from build123d import *

# Parameters (mm, degrees)
SKETCH_1_W                       = 78
SKETCH_1_H                       = 20
SM_BASE_FLANGE_1_DEPTH           = 1.5
SM_EDGE_FLANGE_1_STRIP_W         = 7.4732
SM_EDGE_FLANGE_1_STRIP_H         = 1.5
SM_EDGE_FLANGE_1_STRIP_CUT_DEPTH = 20
SM_EDGE_FLANGE_1_DEPTH           = 20
SM_EDGE_FLANGE_2_STRIP_W         = 7.4732
SM_EDGE_FLANGE_2_STRIP_H         = 1.5
SM_EDGE_FLANGE_2_STRIP_CUT_DEPTH = 20
SM_EDGE_FLANGE_2_DEPTH           = 20


# Sheet-metal steps are written as plain solids
with BuildPart() as part:
    # Sketch 1 → Базовая кромка1 (new body)
    with BuildSketch(Plane(origin=(0, 0, 0), x_dir=(1, 0, 0), z_dir=(0, 1, 0))):
        with Locations((39, 10)):
            Rectangle(SKETCH_1_W, SKETCH_1_H)
    extrude(amount=-SM_BASE_FLANGE_1_DEPTH)

    # Ребро-кромка1 strip (across the edge) → Ребро-кромка1 strip cut (cut)
    with BuildSketch(Plane.XY.offset(-20)):
        with Locations((-1.5, -0.75)):
            Rectangle(SM_EDGE_FLANGE_1_STRIP_W, SM_EDGE_FLANGE_1_STRIP_H)
    extrude(amount=SM_EDGE_FLANGE_1_STRIP_CUT_DEPTH, mode=Mode.SUBTRACT)

    # Ребро-кромка1 section (across the edge) → Ребро-кромка1 (add)
    with BuildSketch(Plane.XY.offset(-20)):
        with BuildLine():
            Line((0, 0.7366), (0, 35))
            Line((0, 35), (1.5, 35))
            Line((1.5, 35), (1.5, 0.7366))
            ThreePointArc((1.5, 0.7366), (1.715745145, 0.215745145), (2.2366, 0))
            Line((2.2366, 0), (2.2366, -1.5))
            ThreePointArc((2.2366, -1.5), (0.655084973, -0.844915027), (0, 0.7366))
        make_face()
    extrude(amount=SM_EDGE_FLANGE_1_DEPTH)

    # Ребро-кромка2 strip (across the edge) → Ребро-кромка2 strip cut (cut)
    with BuildSketch(Plane(origin=(78, 0, 0), x_dir=(-1, 0, 0), z_dir=(0, 0, -1))):
        with Locations((-1.5, -0.75)):
            Rectangle(SM_EDGE_FLANGE_2_STRIP_W, SM_EDGE_FLANGE_2_STRIP_H)
    extrude(amount=SM_EDGE_FLANGE_2_STRIP_CUT_DEPTH, mode=Mode.SUBTRACT)

    # Ребро-кромка2 section (across the edge) → Ребро-кромка2 (add)
    with BuildSketch(Plane(origin=(78, 0, 0), x_dir=(-1, 0, 0), z_dir=(0, 0, -1))):
        with BuildLine():
            Line((0, 0.7366), (0, 35))
            Line((0, 35), (1.5, 35))
            Line((1.5, 35), (1.5, 0.7366))
            ThreePointArc((1.5, 0.7366), (1.715745145, 0.215745145), (2.2366, 0))
            Line((2.2366, 0), (2.2366, -1.5))
            ThreePointArc((2.2366, -1.5), (0.655084973, -0.844915027), (0, 0.7366))
        make_face()
    extrude(amount=SM_EDGE_FLANGE_2_DEPTH)


solid = part.part
The model under review builds one solid part; all positions refer to its coordinate system, in mm. A direction names the side the tool comes from. Round coordinates to 2 decimals unless told otherwise and drop trailing zeros. Order: outer loops, then holes, each group sorted by start corner. A loop starts at its lowest first (then second) coordinate and runs counter-clockwise, first axis right, second up. Notation, with made-up numbers: (87, 84.25) -> (121, 84.25) arc R18 cw to (121, 99.25) -> close; hole circle Ø4 at (2.25, 37). An arc over 180 degrees is marked (long way). Write item = value, one per line. Start each with the question number.
Item 1: Consider section C-C on x = 68.5. Write out the cut boundary in (y, z).
Item 2: Consider section B-B on z = -18. Write out the cut boundary in (x, y), plus the area to 3 significant figures.
Item 3: Mouldability with a two-part tool opening along X and no side actions: class faces 3 (the face through (1.5, 18, -10)), 4 (the face through (1, 35, -10)), 5 (the face through (0.67, -0.86, -10.14)), 6 (the face through (78, 18, -10)) as released by +X, released by -X, zero draft, split by the parting line, or undercut.
Item 4: For line 1 along X through (y, z) = (30, -8.75); line 2 along Y through (x, z) = (35, -8.75), list the stretches that pass through material, from the lowest coordinate up.
Item 5: Consider section A-A on y = 32.5. Write out the cut boundary in (x, z), plus the area to 3 significant figures.
Item 6: For faces 1 (the face through (38, 0, -10)), 2 (the face through (21, -1, -20)), list the 3-axis set-ups (+Z, -Z, +X, -X, +Y, -Y) from which the entire face can be reached by the end or side of a thin tool; tool diameter is ignored.
Item 7: Clearance check with flat-ended pins moving along their axes: pin 1 Ø12 at (x, z) = (35, -8) entering from +Y; pin 2 Ø4 at (y, z) = (14.5, -10) entering from -X. State where each tip first meets the part, or that it passes through.
Conclusion:
q1.outline = (-1.5, -20) -> (0, -20) -> (0, 0) -> (-1.5, 0) -> close
q2.outline = (0, 0.74) arc R2.24 ccw to (2.24, -1.5) -> (75.76, -1.5) arc R2.24 ccw to (78, 0.74) -> (78, 35) -> (76.5, 35) -> (76.5, 0.74) arc R0.74 cw to (75.76, 0) -> (2.24, 0) arc R0.74 cw to (1.5, 0.74) -> (1.5, 35) -> (0, 35) -> close
q2.area = 220 mm2
q3.face_3 = undercut
q3.face_4 = zero draft
q3.face_5 = released by -X
q3.face_6 = released by +X
q4.line_1 = 0 to 1.5, 76.5 to 78
q4.line_2 = -1.5 to 0
q5.outline = (0, -20) -> (1.5, -20) -> (1.5, 0) -> (0, 0) -> close; (76.5, -20) -> (78, -20) -> (78, 0) -> (76.5, 0) -> close
q5.area = 60.0 mm2
q6.face_1 = +Z, -Z, +Y
q6.face_2 = -Z, +X, -X, +Y, -Y
q7.pin_1 = 0
q7.pin_2 = 0
